Answer from the drawing. Dimensions are ordinates in mm from the lowest x, y and z of the part. A direction names the side the tool comes from. Give positions to 0.01 mm unless a question says otherwise; leave off trailing zeros. Order: outer loops, then holes, each group sorted by start corner. A loop starts at its lowest first (then second) coordinate and runs counter-clockwise, first axis right, second up.
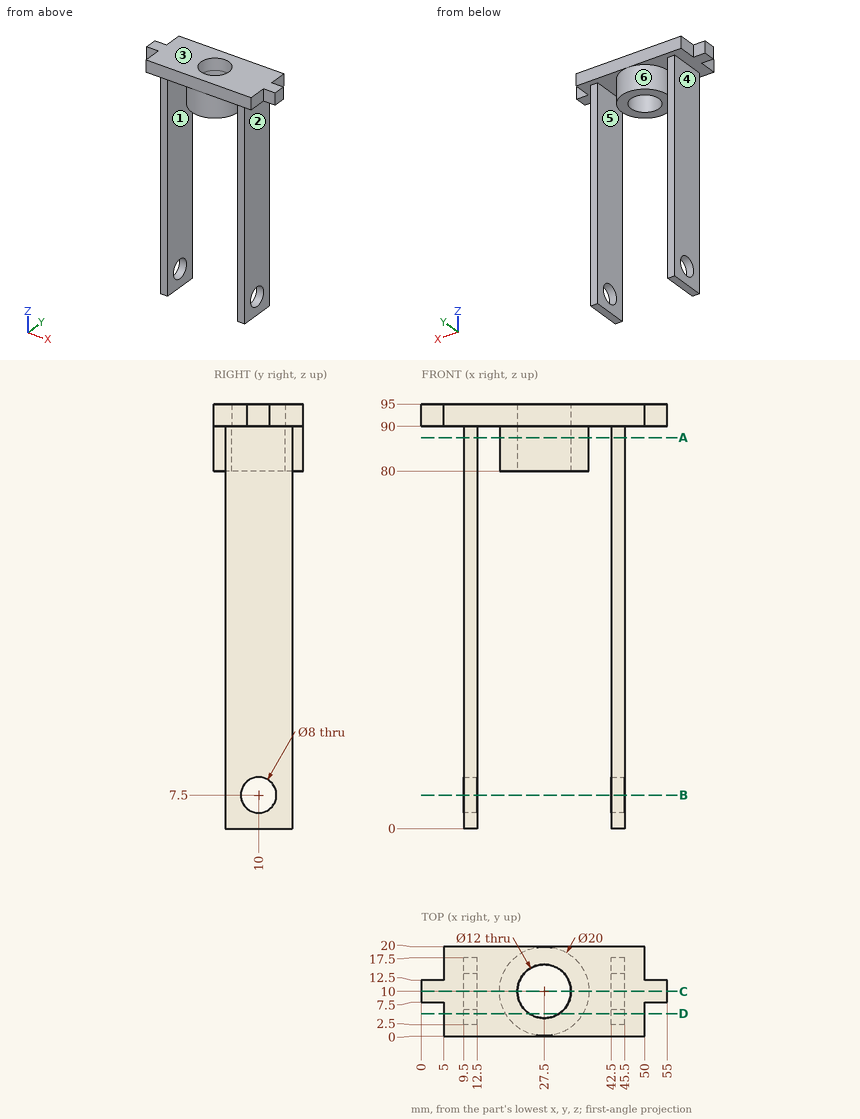
1) The part is cut by section D-D on y = 5. Determine the outline of the cut face in (x, z).
Final values:
outline: (5, 90) - (9.5, 90) - (9.5, 0) - (12.5, 0) - (12.5, 90) - (18.84, 90) - (18.84, 80) - (24.18, 80) - (24.18, 95) - (5, 95) - close; (30.82, 80) - (36.16, 80) - (36.16, 90) - (42.5, 90) - (42.5, 0) - (45.5, 0) - (45.5, 90) - (50, 90) - (50, 95) - (30.82, 95) - close
2) For a pull along X with two mould halves and no side action, classify the marked faces 1, 2, 3 and 4 as released by +X, released by -X, zero draft, split by the parting line, or undercut.
Final values:
face 1: undercut
face 2: released by +X
face 3: zero draft
face 4: released by -X
3) The part is cut by section A-A on z = 87.5. Determine the outline of the cut face in (x, y).
Final values:
outline: (9.5, 2.5) - (12.5, 2.5) - (12.5, 17.5) - (9.5, 17.5) - close; circle Ø20 at (27.5, 10); (42.5, 2.5) - (45.5, 2.5) - (45.5, 17.5) - (42.5, 17.5) - close; hole circle Ø12 at (27.5, 10)
4) Given pin 1 (7.5 mm diameter, centred on y = 12.5, z = 65.5, fed in from +X); pin 2 (2 mm diameter, centred on x = 47.5, z = 79, fed in from +Y); pin 3 (1 mm diameter, centred on x = 16, y = 16, fed in from -Z); pin 4 (8 mm diameter, centred on x = 6, z = 73.5, fed in from -Y), each flat-ended and moving along its own axis, determine where each tip first touches the part or whether it passes through.
Final values:
pin 1: stops at x = 45.5
pin 2: passes through
pin 3: stops at z = 90
pin 4: stops at y = 2.5
5) The part is cut by section C-C on y = 10. Determine the outline of the cut face in (x, z).
Final values:
outline: (0, 90) - (9.5, 90) - (9.5, 11.5) - (12.5, 11.5) - (12.5, 90) - (17.5, 90) - (17.5, 80) - (21.5, 80) - (21.5, 95) - (0, 95) - close; (9.5, 0) - (12.5, 0) - (12.5, 3.5) - (9.5, 3.5) - close; (33.5, 80) - (37.5, 80) - (37.5, 90) - (42.5, 90) - (42.5, 11.5) - (45.5, 11.5) - (45.5, 90) - (55, 90) - (55, 95) - (33.5, 95) - close; (42.5, 0) - (45.5, 0) - (45.5, 3.5) - (42.5, 3.5) - close
6) A tool of negligible diameter and unlimited length cuts with its end or side. For the marked faces 5 and 6, from which of +Z, -Z, +X, -X, +Y, -Y can it reach the whole face along a straight path? Write none if from no direction.
Final values:
face 5: -Z, +Y, -Y
face 6: -Z
7) Consider L1, parallel to X at y = 7, z = 18; L2, parallel to Y at x = 43.9, z = 7.5; L3, parallel to X at y = 8.75, z = 81. Determine where each line is inside the solid, lowest interval first.
Final values:
L1: x = 9.5 to 12.5, 42.5 to 45.5
L2: y = 2.5 to 6, 14 to 17.5
L3: x = 9.5 to 12.5, 17.58 to 21.63, 33.37 to 37.42, 42.5 to 45.5
8) The part is cut by section B-B on z = 7.5. Determine the outline of the cut face in (x, y).
Final values:
outline: (9.5, 2.5) - (12.5, 2.5) - (12.5, 6) - (9.5, 6) - close; (9.5, 14) - (12.5, 14) - (12.5, 17.5) - (9.5, 17.5) - close; (42.5, 2.5) - (45.5, 2.5) - (45.5, 6) - (42.5, 6) - close; (42.5, 14) - (45.5, 14) - (45.5, 17.5) - (42.5, 17.5) - close
